The model under review builds one solid part; all positions refer to its coordinate system, in mm. A direction names the side the tool comes from. Give positions to 0.01 mm unless a question says otherwise; leave off trailing zeros. Order: outer loops, then holes, each group sorted by start corner. A loop starts at its lowest first (then second) coordinate and runs counter-clockwise, first axis right, second up.
```python
from build123d import *

# Parameters (mm, degrees)
SKETCH_1_W            = 88.5
SKETCH_1_H            = 96
SKETCH_1_W_2          = 51.5
SKETCH_1_H_2          = 70.5
SKETCH_1_W_3          = 19
SKETCH_1_H_3          = 71
EXTRUDE_1_DEPTH       = 9.5
SKETCH_5_W            = 88.5
SKETCH_5_H            = 96
EXTRUDE_4_DEPTH       = 4
SKETCH_6_W            = 51.5
SKETCH_6_H            = 1
EXTRUDE_6_DEPTH       = 4
FILLET_3_R            = 9.5
SKETCH_7_W            = 8
SKETCH_7_H            = 9.5
SKETCH_7_W_2          = 37
SKETCH_7_H_2          = 1.5
CUT_EXTRUDE_1_DEPTH   = 4.5
SKETCH_8_W            = 2.5
SKETCH_8_H            = 30
CUT_EXTRUDE_2_DEPTH   = 5.5
SKETCH_9_W            = 19
SKETCH_9_H            = 4.5
EXTRUDE_7_DEPTH       = 9.5
FILLET_4_R            = 9.5
CUT_EXTRUDE_3_DEPTH   = 2.5
SKETCH_11_R           = 3.75
CUT_EXTRUDE_4_DEPTH   = 2.5
SKETCH_13_R           = 1.7
CUT_EXTRUDE_5_DEPTH   = 73.573120111
SKETCH_14_R           = 1.7
CUT_EXTRUDE_6_DEPTH   = 73.573120111
CHAMFER_1_SIZE        = 1.5
SKETCH_15_W           = 6
SKETCH_15_H           = 71
CUT_EXTRUDE_7_DEPTH   = 9.5
CUT_EXTRUDE_9_REACH   = 82.165
SKETCH_18_W           = 2.9
SKETCH_18_H           = 7.825684219
CUT_EXTRUDE_10_DEPTH  = 2.5
SKETCH_19_W           = 3.75
SKETCH_19_H           = 9.5
CUT_EXTRUDE_11_DEPTH  = 2.5
FILLET_5_R            = 3
CUT_EXTRUDE_2_2_DEPTH = 3
EXTRUDE_8_DEPTH       = 4
FILLET_6_R            = 3


with BuildPart() as part:
    # Эскиз1 → Бобышка-Вытянуть1 (new body)
    with BuildSketch(Plane(origin=(0, 0, 0), x_dir=(1, 0, 0), z_dir=(0, 1, 0))):
        with Locations((-4.541472233, 4)):
            Rectangle(SKETCH_1_W, SKETCH_1_H)
        with Locations((5.958527767, -0.75)):
            Rectangle(SKETCH_1_W_2, SKETCH_1_H_2, mode=Mode.SUBTRACT)
        with Locations((-31.291472233, 4)):
            Rectangle(SKETCH_1_W_3, SKETCH_1_H_3, mode=Mode.SUBTRACT)
    extrude(amount=EXTRUDE_1_DEPTH)

    # Эскиз5 → Бобышка-Вытянуть4 (add)
    with BuildSketch(Plane(origin=(0, 9.5, 0), x_dir=(1, 0, 0), z_dir=(0, 1, 0))):
        with Locations((-4.541472233, 4)):
            Rectangle(SKETCH_5_W, SKETCH_5_H)
    extrude(amount=EXTRUDE_4_DEPTH)

    # Эскиз6 → Бобышка-Вытянуть6 (add)
    with BuildSketch(Plane.XZ.offset(-9.5)):
        with Locations((5.958527767, 35.5)):
            Rectangle(SKETCH_6_W, SKETCH_6_H)
        with Locations((5.958527767, -34)):
            Rectangle(SKETCH_6_W, SKETCH_6_H)
    extrude(amount=EXTRUDE_6_DEPTH)

    # Скругление3
    fillet_3_edges = [part.edges().sort_by_distance(p)[0] for p in [
        (-40.791472233, 9.5, -4),
        (-21.791472233, 9.5, -4),
    ]]
    fillet(fillet_3_edges, radius=FILLET_3_R - 0.0001)  # a hair under: the kernel refuses the full size

    # Эскиз7 → Вырез-Вытянуть1 (cut)
    with BuildSketch(Plane.XZ):
        with Locations((27.708527767, -39.25)):
            Rectangle(SKETCH_7_W, SKETCH_7_H)
        with Locations((-1.291472233, -35.25)):
            Rectangle(SKETCH_7_W_2, SKETCH_7_H_2)
    extrude(amount=-CUT_EXTRUDE_1_DEPTH, mode=Mode.SUBTRACT)

    # Эскиз8 → Cut-Extrude 2 (cut)
    with BuildSketch(Plane.XZ):
        with Locations((32.958527767, 21)):
            Rectangle(SKETCH_8_W, SKETCH_8_H)
    extrude(amount=-CUT_EXTRUDE_2_DEPTH, mode=Mode.SUBTRACT)

    # Эскиз9 → Бобышка-Вытянуть7 (add)
    with BuildSketch(Plane.XZ):
        with Locations((-31.291472233, 33.75)):
            Rectangle(SKETCH_9_W, SKETCH_9_H)
        with Locations((-31.291472233, -41.75)):
            Rectangle(SKETCH_9_W, SKETCH_9_H)
    extrude(amount=EXTRUDE_7_DEPTH)

    # Скругление4
    fillet_4_edges = [part.edges().sort_by_distance(p)[0] for p in [
        (-21.791472233, -9.5, 33.75),
        (-21.791472233, -9.5, -41.75),
        (-40.791472233, -9.5, -41.75),
        (-40.791472233, -9.5, 33.75),
    ]]
    fillet(fillet_4_edges, radius=FILLET_4_R - 0.0001)  # a hair under: the kernel refuses the full size

    # Эскиз10 → Вырез-Вытянуть3 (cut)
    with BuildSketch(Plane(origin=(0, 0, 31.5), x_dir=(-1, 0, 0), z_dir=(0, 0, -1))):
        Polygon((31.291472233, 3.348631561), (28.391472233, 1.674315781), (28.391472233, -1.674315781), (31.291472233, -3.348631561), (34.191472233, -1.674315781), (34.191472233, 1.674315781), align=None)
    extrude(amount=-CUT_EXTRUDE_3_DEPTH, mode=Mode.SUBTRACT)

    # Эскиз11 → Вырез-Вытянуть4 (cut)
    with BuildSketch(Plane.XY.offset(-39.5)):
        with Locations((-31.291472233, 0)):
            Circle(SKETCH_11_R)
    extrude(amount=-CUT_EXTRUDE_4_DEPTH, mode=Mode.SUBTRACT)

    # Эскиз13 → Вырез-Вытянуть5 (cut, through all)
    with BuildSketch(Plane.XZ):
        with Locations(Location((35.308527767, 39.6, 0), (0, 0, 90))):
            Circle(SKETCH_13_R)
        with Locations(Location((-44.391472233, 39.6, 0), (0, 0, 270))):
            Circle(SKETCH_13_R)
        with Locations(Location((-44.391472233, -47.6, 0), (0, 0, 90))):
            Circle(SKETCH_13_R)
        with Locations(Location((35.308527767, -47.6, 0), (0, 0, 270))):
            Circle(SKETCH_13_R)
    extrude(amount=-CUT_EXTRUDE_5_DEPTH, mode=Mode.SUBTRACT)

    # Эскиз14 → Вырез-Вытянуть6 (cut, through all)
    with BuildSketch(Plane.XZ):
        with Locations(Location((-4.541472233, -47.6, 0), (0, 0, 270))):
            Circle(SKETCH_14_R)
        with Locations(Location((-4.541472233, 39.6, 0), (0, 0, 90))):
            Circle(SKETCH_14_R)
        with Locations(Location((-44.391472233, -4, 0), (0, 0, 270))):
            Circle(SKETCH_14_R)
        with Locations(Location((35.308527767, -4, 0), (0, 0, 90))):
            Circle(SKETCH_14_R)
    extrude(amount=-CUT_EXTRUDE_6_DEPTH, mode=Mode.SUBTRACT)

    # Фаска1
    chamfer_1_edges = [part.edges().sort_by_distance(p)[0] for p in [
        (-44.391472233, 13.5, 41.3),
        (35.308527767, 13.5, 37.9),
        (-44.391472233, 13.5, -49.3),
        (35.308527767, 13.5, -45.9),
        (-4.541472233, 13.5, -45.9),
        (-4.541472233, 13.5, 37.9),
        (-44.391472233, 13.5, -2.3),
        (35.308527767, 13.5, -5.7),
    ]]
    chamfer(chamfer_1_edges, length=CHAMFER_1_SIZE)

    # Эскиз15 → Вырез-Вытянуть7 (cut)
    with BuildSketch(Plane.XZ):
        with Locations((-28.291472233, -4)):
            Rectangle(SKETCH_15_W, SKETCH_15_H)
    extrude(amount=-CUT_EXTRUDE_7_DEPTH, mode=Mode.SUBTRACT)

    # Вырез-Вытянуть9: up to this face of the body (flat: up to its plane)
    cut_extrude_9_end = Plane(part.part.faces().sort_by_distance((-25.291472233, 8.432756206, -4))[0])
    # Эскиз17 → Вырез-Вытянуть9 (cut, up to the picked face)
    with BuildSketch(Plane(origin=(-19.791472233, 0, 0), x_dir=(0, 0, -1), z_dir=(1, 0, 0)), mode=Mode.PRIVATE) as cut_extrude_9_sk1:
        with BuildLine():
            Line((-31.5, 9.5), (-26.5, 9.5))
            Line((-26.5, 9.5), (-26.5, 6.283345014))
            ThreePointArc((-26.5, 6.283345014), (-27.085786438, 4.869131452), (-28.5, 4.283345014))
            Line((-28.5, 4.283345014), (-29.5, 4.283345014))
            ThreePointArc((-29.5, 4.283345014), (-30.914213562, 4.869131452), (-31.5, 6.283345014))
            Line((-31.5, 6.283345014), (-31.5, 9.5))
        make_face()
    cut_extrude_9_tool1 = split(extrude(cut_extrude_9_sk1.sketch, amount=-CUT_EXTRUDE_9_REACH, mode=Mode.PRIVATE), bisect_by=cut_extrude_9_end, keep=Keep.BOTH, mode=Mode.PRIVATE)
    add(cut_extrude_9_tool1.solids().sort_by(Axis((-19.791472, 7.043974, 29), (-1, 0, 0)))[0], mode=Mode.SUBTRACT)

    # Эскиз18 → Вырез-Вытянуть10 (cut)
    with BuildSketch(Plane(origin=(0, 0, 31.5), x_dir=(-1, 0, 0), z_dir=(0, 0, -1))):
        with Locations((29.841472233, 5.587157891)):
            Rectangle(SKETCH_18_W, SKETCH_18_H)
    extrude(amount=-CUT_EXTRUDE_10_DEPTH, mode=Mode.SUBTRACT)

    # Эскиз19 → Вырез-Вытянуть11 (cut)
    with BuildSketch(Plane.XY.offset(-39.5)):
        with Locations((-29.416472233, 4.75)):
            Rectangle(SKETCH_19_W, SKETCH_19_H)
    extrude(amount=-CUT_EXTRUDE_11_DEPTH, mode=Mode.SUBTRACT)

    # Скругление5
    fillet_5_edges = [part.edges().sort_by_distance(p)[0] for p in [
        (-48.791472233, 6.75, -52),
        (39.708527767, 6.75, -52),
        (39.708527767, 6.75, 44),
        (-48.791472233, 6.75, 44),
    ]]
    fillet(fillet_5_edges, radius=FILLET_5_R)

    # Эскиз21 → Cut-Extrude 2 2 (cut)
    with BuildSketch(Plane.XZ):
        with BuildLine():
            Line((-48.791472233, -49), (-48.791472233, 41))
            ThreePointArc((-48.791472233, 41), (-47.912792577, 43.121320344), (-45.791472233, 44))
            Line((-45.791472233, 44), (36.708527767, 44))
            ThreePointArc((36.708527767, 44), (38.82984811, 43.121320344), (39.708527767, 41))
            Line((39.708527767, 41), (39.708527767, -49))
            ThreePointArc((39.708527767, -49), (38.82984811, -51.121320344), (36.708527767, -52))
            Line((36.708527767, -52), (-45.791472233, -52))
            ThreePointArc((-45.791472233, -52), (-47.912792577, -51.121320344), (-48.791472233, -49))
        make_face()
        with BuildLine():
            Line((-47.291472233, -49), (-47.291472233, 41))
            ThreePointArc((-47.291472233, 41), (-46.852132405, 42.060660172), (-45.791472233, 42.5))
            Line((-45.791472233, 42.5), (36.708527767, 42.5))
            ThreePointArc((36.708527767, 42.5), (37.769187939, 42.060660172), (38.208527767, 41))
            Line((38.208527767, 41), (38.208527767, -49))
            ThreePointArc((38.208527767, -49), (37.769187939, -50.060660172), (36.708527767, -50.5))
            Line((36.708527767, -50.5), (-45.791472233, -50.5))
            ThreePointArc((-45.791472233, -50.5), (-46.852132405, -50.060660172), (-47.291472233, -49))
        make_face(mode=Mode.SUBTRACT)
    extrude(amount=-CUT_EXTRUDE_2_2_DEPTH, mode=Mode.SUBTRACT)

    # Эскиз22 → Бобышка-Вытянуть8 (add)
    with BuildSketch(Plane(origin=(0, 13.5, 0), x_dir=(1, 0, 0), z_dir=(0, 1, 0))):
        with BuildLine():
            Line((-48.791472233, -6), (-51.791472233, -6))
            ThreePointArc((-51.791472233, -6), (-53.205685795, -5.414213562), (-53.791472233, -4))
            Line((-53.791472233, -4), (-53.791472233, 12))
            ThreePointArc((-53.791472233, 12), (-53.205685795, 13.414213562), (-51.791472233, 14))
            Line((-51.791472233, 14), (-48.791472233, 14))
            Line((-48.791472233, 14), (-48.791472233, 20))
            Line((-48.791472233, 20), (-57.791472233, 20))
            ThreePointArc((-57.791472233, 20), (-59.205685795, 19.414213562), (-59.791472233, 18))
            Line((-59.791472233, 18), (-59.791472233, -10))
            ThreePointArc((-59.791472233, -10), (-59.205685795, -11.414213562), (-57.791472233, -12))
            Line((-57.791472233, -12), (-48.791472233, -12))
            Line((-48.791472233, -12), (-48.791472233, -6))
        make_face()
        with BuildLine():
            Line((39.708527767, -6), (39.708527767, -12))
            Line((39.708527767, -12), (48.708527767, -12))
            ThreePointArc((48.708527767, -12), (50.122741329, -11.414213562), (50.708527767, -10))
            Line((50.708527767, -10), (50.708527767, 18))
            ThreePointArc((50.708527767, 18), (50.122741329, 19.414213562), (48.708527767, 20))
            Line((48.708527767, 20), (39.708527767, 20))
            Line((39.708527767, 20), (39.708527767, 14))
            Line((39.708527767, 14), (42.708527767, 14))
            ThreePointArc((42.708527767, 14), (44.122741329, 13.414213562), (44.708527767, 12))
            Line((44.708527767, 12), (44.708527767, -4))
            ThreePointArc((44.708527767, -4), (44.122741329, -5.414213562), (42.708527767, -6))
            Line((42.708527767, -6), (39.708527767, -6))
        make_face()
    extrude(amount=-EXTRUDE_8_DEPTH)

    # Скругление6
    fillet_6_edges = [part.edges().sort_by_distance(p)[0] for p in [
        (-48.791472233, 11.5, -14),
        (-48.791472233, 11.5, 6),
        (-48.791472233, 11.5, -20),
        (-48.791472233, 11.5, 12),
        (39.708527767, 11.5, 6),
        (39.708527767, 11.5, -14),
        (39.708527767, 11.5, 12),
        (39.708527767, 11.5, -20),
    ]]
    fillet(fillet_6_edges, radius=FILLET_6_R - 0.0001)  # a hair under: the kernel refuses the full size


solid = part.part
```
1. Draft analysis for pull direction Z (two halves, no side actions). For faces 1 (the cylindrical face through (38.81, 8.32, 43.14)), 2 (the flat face through (-47.291, 1, -5)), 3 (the cylindrical face through (-45.04, 5.92, -5.57)), state which applies: pulls with the +Z half, pulls with the -Z half, needs draft (parallel to the pull), parting line crosses it, or undercut.
2. Insertion check: pin 1 (4 mm diameter, centred on x = 35.31, z = -47.6, fed in from +Y); pin 2 (5 mm diameter, centred on y = 3.5, z = 0, fed in from -X); pin 3 (2 mm diameter, centred on y = 5.5, z = -14.5, fed in from +X); pin 4 (2 mm diameter, centred on x = -44.39, z = -4, fed in from -Y). Each pin has a flat end and moves straight along its axis. Give the tip position at first contact, or say it passes through.
3. To check wall thickness, follow line 1 (X direction, y = 9.5, z = 39.6); line 2 (X direction, y = 0.25, z = -2); line 3 (X direction, y = 6.75, z = 33). State the ranges of each line that lie inside material, in increasing order.
4. Take a section at C-C (y = -5). Write out the cut boundary in (x, z), and give its area (3 significant figures).
5. Take a section at A-A (z = -47.6). Write out the cut boundary in (x, y), and give its area (3 significant figures).
6. For faces 4 (the flat face through (46, 12, -20)), 5 (the flat face through (-23, 8, 26.5)), 6 (the flat face through (-2, 2, -36)), 7 (the cylindrical face through (40.564, 11.472, 5.098)), list the 3-axis set-ups (+Z, -Z, +X, -X, +Y, -Y) from which the entire face can be reached by the end or side of a thin tool; tool diameter is ignored.
7. Take a section at B-B (x = -13). Write out the cut boundary in (y, z), and give its area (4 significant figures).
Answer:
1. face 1: pulls with the +Z half
1. face 2: needs draft
1. face 3: undercut
2. pin 1: stops at y = 12.3
2. pin 2: stops at x = -48.79
2. pin 3: stops at x = 39.71
2. pin 4: passes through
3. line 1: x = -48.79 to -46.09, -42.69 to -6.24, -2.84 to 33.61, 37.01 to 39.71
3. line 2: x = -47.29 to -40.79, -21.79 to -19.79, 31.71 to 38.21
3. line 3: x = -48.79 to -31.29, -28.39 to -19.79, 31.71 to 39.71
4. outline: (-39.37, -44) - (-23.21, -44) - (-23.21, -39.5) - (-39.37, -39.5) - close; (-39.37, 31.5) - (-23.21, 31.5) - (-23.21, 36) - (-39.37, 36) - close
4. area: 145 mm2
5. outline: (-48.79, 3) - (-47.29, 3) - (-47.29, 0) - (-46.09, 0) - (-46.09, 12) - (-47.59, 13.5) - (-48.79, 13.5) - close; (-42.69, 0) - (-6.24, 0) - (-6.24, 12) - (-7.74, 13.5) - (-41.19, 13.5) - (-42.69, 12) - close; (-2.84, 0) - (33.61, 0) - (33.61, 12) - (32.11, 13.5) - (-1.34, 13.5) - (-2.84, 12) - close; (37.01, 0) - (38.21, 0) - (38.21, 3) - (39.71, 3) - (39.71, 13.5) - (38.51, 13.5) - (37.01, 12) - close
5. area: 1,040 mm2
6. face 4: -Z, +X, +Y, -Y
6. face 5: none
6. face 6: -Y
6. face 7: +Y, -Y
7. outline: (0, -50.5) - (3, -50.5) - (3, -52) - (13.5, -52) - (13.5, 44) - (3, 44) - (3, 42.5) - (0, 42.5) - (0, 36) - (5.5, 36) - (5.5, 35) - (9.5, 35) - (9.5, -33.5) - (5.5, -33.5) - (5.5, -34.5) - (4.5, -34.5) - (4.5, -36) - (0, -36) - close
7. area: 618.5 mm2
